The listing builds one solid part. Answer for the finished solid, in the listing's coordinates (mm). Face numbers are marked on the shaded views. A direction names the side the tool comes from. Round coordinates to 2 decimals unless told otherwise and drop trailing zeros. Loops run counter-clockwise (first coordinate to the right, second up) from the corner with the lowest first, then second, coordinate; pieces in that order, holes last. Notation, with made-up numbers: M -11.5,23 L 45.5,23 A14 ccw 45.5,32 Z; hole C 4.5,63.5 d6. An arc over 180 degrees is marked long. Answer as a JSON object with one key per item and string values.
```python
from build123d import *

# Parameters (mm, degrees)
SKETCH_W        = 45
SKETCH_H        = 37.5
PAD_DEPTH       = 20
POCKET_DEPTH    = 18
SKETCH002_R     = 1.3
POCKET003_DEPTH = 15
SKETCH003_W     = 6
SKETCH003_H     = 2.6407929057
POCKET001_DEPTH = 3
PAD002_DEPTH    = 45


with BuildPart() as part:
    # Sketch → Pad (new body)
    with BuildSketch(Plane.XY):
        Rectangle(SKETCH_W, SKETCH_H)
    extrude(amount=PAD_DEPTH)

    # Sketch001 (on Face6 of Pad) → Pocket (cut)
    with BuildSketch(Plane.XY.offset(20)):
        with BuildLine():
            Line((8.5, 10.6092070943), (8.5, 16.1092070943))
            Line((8.5, 16.1092070943), (-8.5, 16.1092070943))
            Line((-8.5, 16.1092070943), (-8.5, 10.6092070943))
            ThreePointArc((-8.5, 10.6092070943), (0, -16.75), (8.5, 10.6092070943))
        make_face()
    extrude(amount=-POCKET_DEPTH, mode=Mode.SUBTRACT)

    # Sketch002 (on Face5 of Pocket) → Pocket003 (cut)
    with BuildSketch(Plane.XY.offset(20)):
        with Locations((-17.25, -1)):
            Circle(SKETCH002_R)
        with Locations((17.25, -1)):
            Circle(SKETCH002_R)
    extrude(amount=-POCKET003_DEPTH, mode=Mode.SUBTRACT)

    # Sketch003 (on Face5 of Pocket003) → Pocket001 (cut)
    with BuildSketch(Plane.XY.offset(20)):
        with Locations((0, 17.4296035472)):
            Rectangle(SKETCH003_W, SKETCH003_H)
    extrude(amount=-POCKET001_DEPTH, mode=Mode.SUBTRACT)

    # Sketch006 (on Face8 of Pocket001) → Pad002 (join)
    with BuildSketch(Plane(origin=(-22.5, 0, 0), x_dir=(0, -1, 0), z_dir=(-1, 0, 0))):
        with BuildLine():
            ThreePointArc((47.2114813968, 16.5), (21.25, 15.5), (47.2114813968, 14.5))
            Line((61.25, 14.5), (47.2114813968, 14.5))
            Line((61.25, 12), (61.25, 14.5))
            Line((49.3496688705, 12), (61.25, 12))
            ThreePointArc((34.2500364402, 0), (43.8936650252, 3.3653502365), (49.3496688705, 12))
            Line((18.75, 0), (34.2500364402, 0))
            Line((18.75, 0), (18.75, 20))
            Line((18.75, 20), (19.4176030258, 20))
            ThreePointArc((49.3496688705, 19), (34.767550545, 30.9913569913), (19.4176030258, 20))
            Line((61.25, 19), (49.3496688705, 19))
            Line((61.25, 16.5), (61.25, 19))
            Line((47.2114813968, 16.5), (61.25, 16.5))
        make_face()
    extrude(amount=-PAD002_DEPTH)


solid = part.part
```
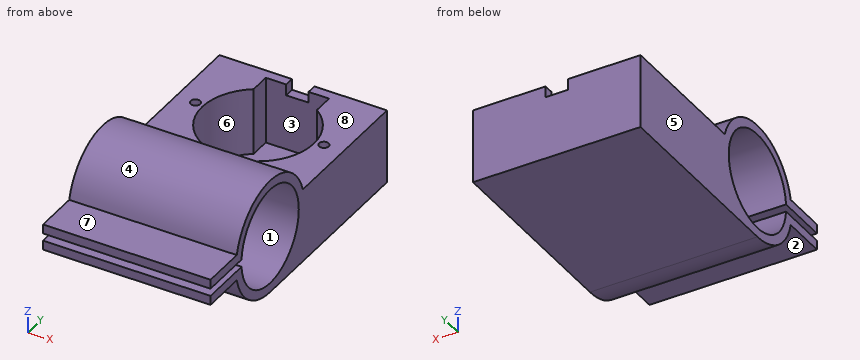
Item 1: Determine the mould class of the marked faces 1, 2, 3 and 4 for opening direction Z: released by +Z, released by -Z, zero draft, split by the parting line, or undercut.
Values follow:
{"face 1": "undercut", "face 2": "released by -Z", "face 3": "zero draft", "face 4": "released by +Z"}
Item 2: Straight lines are drawn through the part: line 1 (Z direction, x = -11.5, y = -51.5); line 2 (Z direction, x = 3, y = -34); line 3 (X direction, y = 12, z = 8.5). For each, find the intervals that lie inside material, in ascending order.
Values follow:
{"line 1": "12 to 14.5, 16.5 to 19", "line 2": "0 to 2.5, 28.5 to 31", "line 3": "-22.5 to -8.5, 8.5 to 22.5"}
Item 3: The part is cut by section A-A (z = 7.5). Give the vertices of the cut face in (x, y).
Values follow:
{"outline": "M -22.5,-47.53 L 22.5,-47.53 L 22.5,-44.5 L -22.5,-44.5 Z; M -22.5,-24 L 22.5,-24 L 22.5,18.75 L -22.5,18.75 Z; hole C -17.25,-1 d2.6; hole M -8.5,10.61 A15 ccw long 8.5,10.61 L 8.5,16.11 L -8.5,16.11 Z; hole C 17.25,-1 d2.6"}
Item 4: Flat-ended cylindrical pins translate along their axes: P1, Ø5, axis at x = 13, y = -47, coming from the +Z side; P2, Ø0.8, axis at x = 18, y = -1, coming from the +Z side; P3, Ø3, axis at x = 10, z = 25.5, coming from the -Y side; P4, Ø4, axis at y = -52, z = 21.5, coming from the -X side. Find the tip coordinate at first contact, or state that the pin passes through.
Values follow:
{"P1": "z = 27.13", "P2": "z = 5", "P3": "y = -47.21", "P4": "through"}
Item 5: The part is cut by section C-C (y = -30). Give the vertices of the cut face in (x, z).
Values follow:
{"outline": "M -22.5,0 L 22.5,0 L 22.5,3.21 L -22.5,3.21 Z; M -22.5,27.79 L 22.5,27.79 L 22.5,30.41 L -22.5,30.41 Z"}
Item 6: Which of the six approach directions +Z, -Z, +X, -X, +Y, -Y give full straight-line access (tool end or side, diameter ignored) to the marked faces 5, 6, 7 and 8?
Values follow:
{"face 5": "+Z, -Z, -X, +Y, -Y", "face 6": "+Z", "face 7": "+Z, +X, -X, -Y", "face 8": "+Z, +X, -X, +Y"}
Item 7: The part is cut by section D-D (z = 21). Give the vertices of the cut face in (x, y).
Values follow:
{"outline": "M -22.5,-48.74 L 22.5,-48.74 L 22.5,-46.03 L -22.5,-46.03 Z; M -22.5,-22.47 L 22.5,-22.47 L 22.5,-19.76 L -22.5,-19.76 Z"}
Item 8: The part is cut by section B-B (x = 0). Give the vertices of the cut face in (y, z).
Values follow:
{"outline": "M -61.25,12 L -49.35,12 A15.5 ccw -34.25,0 L 18.75,0 L 18.75,17 L 16.11,17 L 16.11,2 L -16.75,2 L -16.75,20 L -19.42,20 A15.5 ccw -49.35,19 L -61.25,19 L -61.25,16.5 L -47.21,16.5 A13 cw long -47.21,14.5 L -61.25,14.5 Z"}
